```python
from build123d import *

# Parameters (mm, degrees)
CROQUIS2_R                    = 2.0193
CROQUIS2_R_2                  = 14.3256
CROQUIS2_R_3                  = 2.4892
SALIENTE_EXTRUIR1_DEPTH       = 6.35
CROQUIS4_R                    = 11.1125
CROQUIS4_R_2                  = 2.0193
CROQUIS4_R_3                  = 14.3256
CROQUIS4_R_4                  = 2.4892
CROQUIS4_R_5                  = 12.7
SALIENTE_EXTRUIR2_DEPTH       = 6.35
SALIENTE_EXTRUIR3_OUTLINE_R   = 2.4892
SALIENTE_EXTRUIR3_OUTLINE_R_2 = 11.1125
SALIENTE_EXTRUIR3_DEPTH       = 3.175


# Read off the part's stored shape, not the designer's step: Saliente-Extruir3
with BuildPart() as part:
    # Croquis2 → Saliente-Extruir1 (new body)
    with BuildSketch(Plane.XY):
        with BuildLine():
            Line((-50.26025, -3.966971602), (-17.216966667, -25.917547797))
            ThreePointArc((-17.216966667, -25.917547797), (0, -31.115), (17.216966667, -25.917547797))
            Line((17.216966667, -25.917547797), (50.26025, -3.966971602))
            ThreePointArc((50.26025, -3.966971602), (51.383179934, -2.925318757), (52.117388984, -1.581090594))
            Line((52.117388984, -1.581090594), (62.733042527, 28.581409406))
            ThreePointArc((62.733042527, 28.581409406), (59.824949243, 34.653759666), (53.750525482, 31.75))
            ThreePointArc((53.750525482, 31.75), (50.269530675, 27.147870067), (44.770269361, 25.4))
            Line((44.770269361, 25.4), (-44.770269361, 25.4))
            ThreePointArc((-44.770269361, 25.4), (-50.269530675, 27.147870067), (-53.750525482, 31.75))
            ThreePointArc((-53.750525482, 31.75), (-59.824949243, 34.653759666), (-62.733042527, 28.581409406))
            Line((-62.733042527, 28.581409406), (-52.117388984, -1.581090594))
            ThreePointArc((-52.117388984, -1.581090594), (-51.383179934, -2.925318757), (-50.26025, -3.966971602))
        make_face()
        with Locations((23.8125, 0)):
            Circle(CROQUIS2_R, mode=Mode.SUBTRACT)
        with Locations((-23.8125, 0)):
            Circle(CROQUIS2_R, mode=Mode.SUBTRACT)
        Circle(CROQUIS2_R_2, mode=Mode.SUBTRACT)
        with Locations((-47.625, 0)):
            Circle(CROQUIS2_R_3, mode=Mode.SUBTRACT)
        with Locations((47.625, 0)):
            Circle(CROQUIS2_R_3, mode=Mode.SUBTRACT)
        with Locations((-58.240653543, 30.1625)):
            Circle(CROQUIS2_R_3, mode=Mode.SUBTRACT)
        with Locations((58.240653543, 30.1625)):
            Circle(CROQUIS2_R_3, mode=Mode.SUBTRACT)
    extrude(amount=SALIENTE_EXTRUIR1_DEPTH)


with BuildPart() as body_2:
    # Croquis4 → Saliente-Extruir2 (new body)
    with BuildSketch(Plane.XY):
        with BuildLine():
            Line((-63.003153543, 56.9875), (-63.003153543, 30.1625))
            ThreePointArc((-63.003153543, 30.1625), (-62.935140138, 29.360501336), (-62.733042527, 28.581409406))
            Line((-62.733042527, 28.581409406), (-52.117388984, -1.581090594))
            ThreePointArc((-52.117388984, -1.581090594), (-51.383179934, -2.925318757), (-50.26025, -3.966971602))
            Line((-50.26025, -3.966971602), (-17.216966667, -25.917547797))
            ThreePointArc((-17.216966667, -25.917547797), (0, -31.115), (17.216966667, -25.917547797))
            Line((17.216966667, -25.917547797), (50.26025, -3.966971602))
            ThreePointArc((50.26025, -3.966971602), (51.383179934, -2.925318757), (52.117388984, -1.581090594))
            Line((52.117388984, -1.581090594), (62.733042527, 28.581409406))
            ThreePointArc((62.733042527, 28.581409406), (62.935140138, 29.360501336), (63.003153543, 30.1625))
            Line((63.003153543, 30.1625), (63.003153543, 56.9875))
            ThreePointArc((63.003153543, 56.9875), (54.216356978, 78.200703436), (33.003153543, 86.9875))
            Line((33.003153543, 86.9875), (-33.003153543, 86.9875))
            ThreePointArc((-33.003153543, 86.9875), (-54.216356978, 78.200703436), (-63.003153543, 56.9875))
        make_face()
        with Locations((0, 40.64)):
            Circle(CROQUIS4_R, mode=Mode.SUBTRACT)
        with Locations((-16.145831218, -9.3218)):
            Circle(CROQUIS4_R_2, mode=Mode.SUBTRACT)
        Circle(CROQUIS4_R_3, mode=Mode.SUBTRACT)
        with Locations((0, 18.6436)):
            Circle(CROQUIS4_R_2, mode=Mode.SUBTRACT)
        with Locations((16.145831218, -9.3218)):
            Circle(CROQUIS4_R_2, mode=Mode.SUBTRACT)
        with Locations((-47.625, 0)):
            Circle(CROQUIS4_R_4, mode=Mode.SUBTRACT)
        with Locations((47.625, 0)):
            Circle(CROQUIS4_R_4, mode=Mode.SUBTRACT)
        with Locations((-29.02971813, 82.074783851)):
            Circle(CROQUIS4_R_4, mode=Mode.SUBTRACT)
        with Locations((-36.976588955, 31.900216149)):
            Circle(CROQUIS4_R_4, mode=Mode.SUBTRACT)
        with Locations((-33.003153543, 56.9875)):
            Circle(CROQUIS4_R_5, mode=Mode.SUBTRACT)
        with Locations((-58.090437394, 60.960935412)):
            Circle(CROQUIS4_R_4, mode=Mode.SUBTRACT)
        with Locations((-58.240653543, 30.1625)):
            Circle(CROQUIS4_R_4, mode=Mode.SUBTRACT)
        with Locations((58.090437394, 60.960935412)):
            Circle(CROQUIS4_R_4, mode=Mode.SUBTRACT)
        with Locations((36.976588955, 31.900216149)):
            Circle(CROQUIS4_R_4, mode=Mode.SUBTRACT)
        with Locations((33.003153543, 56.9875)):
            Circle(CROQUIS4_R_5, mode=Mode.SUBTRACT)
        with Locations((29.02971813, 82.074783851)):
            Circle(CROQUIS4_R_4, mode=Mode.SUBTRACT)
        with Locations((58.240653543, 30.1625)):
            Circle(CROQUIS4_R_4, mode=Mode.SUBTRACT)
    extrude(amount=-SALIENTE_EXTRUIR2_DEPTH)


with BuildPart() as body_3:
    # Saliente-Extruir3 outline → Saliente-Extruir3 (new body)
    with BuildSketch(Plane.XY):
        with BuildLine():
            Line((-35.881109014, 27.265420582), (-22.987624276, 30.312923688))
            ThreePointArc((-22.987624276, 30.312923688), (-18.059295743, 30.166513899), (-13.86444293, 27.575555036))
            ThreePointArc((-13.86444293, 27.575555036), (0, 21.59), (13.86444293, 27.575555036))
            ThreePointArc((13.86444293, 27.575555036), (18.059295743, 30.166513899), (22.987624276, 30.312923688))
            Line((22.987624276, 30.312923688), (35.881109014, 27.265420582))
            ThreePointArc((35.881109014, 27.265420582), (41.611384522, 30.804736208), (38.072068895, 36.535011716))
            Line((38.072068895, 36.535011716), (23.323178626, 40.021058337))
            ThreePointArc((23.323178626, 40.021058337), (20.26820543, 41.736288231), (18.58786391, 44.81058932))
            ThreePointArc((18.58786391, 44.81058932), (18.032030897, 46.783969542), (17.267348762, 48.686189579))
            ThreePointArc((17.267348762, 48.686189579), (16.412494406, 53.542019269), (18.100083663, 58.174718315))
            Line((18.100083663, 58.174718315), (32.93018787, 79.342066878))
            ThreePointArc((32.93018787, 79.342066878), (31.762435104, 85.975253591), (25.129248391, 84.807500825))
            Line((25.129248391, 84.807500825), (11.314654439, 65.08961339))
            ThreePointArc((11.314654439, 65.08961339), (6.613405383, 61.027851685), (0.54804108, 59.682115192))
            ThreePointArc((0.54804108, 59.682115192), (0, 59.69), (-0.54804108, 59.682115192))
            ThreePointArc((-0.54804108, 59.682115192), (-6.613405383, 61.027851685), (-11.314654439, 65.08961339))
            Line((-11.314654439, 65.08961339), (-25.129248391, 84.807500825))
            ThreePointArc((-25.129248391, 84.807500825), (-31.762435104, 85.975253591), (-32.93018787, 79.342066878))
            Line((-32.93018787, 79.342066878), (-18.100083663, 58.174718315))
            ThreePointArc((-18.100083663, 58.174718315), (-16.412494406, 53.542019269), (-17.267348762, 48.686189579))
            ThreePointArc((-17.267348762, 48.686189579), (-18.032030897, 46.783969542), (-18.58786391, 44.81058932))
            ThreePointArc((-18.58786391, 44.81058932), (-20.26820543, 41.736288231), (-23.323178626, 40.021058337))
            Line((-23.323178626, 40.021058337), (-38.072068895, 36.535011716))
            ThreePointArc((-38.072068895, 36.535011716), (-41.611384522, 30.804736208), (-35.881109014, 27.265420582))
        make_face()
        with Locations((-36.976588955, 31.900216149)):
            Circle(SALIENTE_EXTRUIR3_OUTLINE_R, mode=Mode.SUBTRACT)
        with Locations((36.976588955, 31.900216149)):
            Circle(SALIENTE_EXTRUIR3_OUTLINE_R, mode=Mode.SUBTRACT)
        with Locations((0, 40.64)):
            Circle(SALIENTE_EXTRUIR3_OUTLINE_R_2, mode=Mode.SUBTRACT)
        with Locations((-29.02971813, 82.074783851)):
            Circle(SALIENTE_EXTRUIR3_OUTLINE_R, mode=Mode.SUBTRACT)
        with Locations((29.02971813, 82.074783851)):
            Circle(SALIENTE_EXTRUIR3_OUTLINE_R, mode=Mode.SUBTRACT)
    extrude(amount=SALIENTE_EXTRUIR3_DEPTH)


solid = part.part
```
Design review of the part built by this model. Coordinates are the model's own, in mm. A direction names the side the tool comes from. Give positions to 0.01 mm unless a question says otherwise; leave off trailing zeros. Order: outer loops, then holes, each group sorted by start corner. A loop starts at its lowest first (then second) coordinate and runs counter-clockwise, first axis right, second up. Notation, with made-up numbers: (60.25, 52) -> (65.25, 52) arc R32 ccw to (65.25, 80) -> close; hole circle Ø7 at (86, -23). An arc over 180 degrees is marked (long way). Write each question's results on one line, items separated by ' | '. Start each with the question number.
Q1. Mouldability with a two-part tool opening along X and no side actions: class faces 3 (the flat face through (1, 25.4, 3)), 4 (the cylindrical face through (-59.726, 34.687, 3.131)), 5 (the flat face through (-1, 17, 0)), 6 (the cylindrical face through (-51.396, -2.908, 3.131)) as +X half, -X half, draft (parallel to the pull), parting line (faces both ways), or undercut.
Q2. Add section C-C on y = 0. Give the boundary of the cut face in (x, z).
Q3. Add section A-A on x = 0. Give the boundary of the cut face in (y, z) (3 decimals).
Q4. Add section B-B on y = 12. Give the boundary of the cut face in (x, z), and give its area (3 significant figures).
Q5. Add section D-D on z = 4.75. State how many separate pieces and enclosed holes the cut face has, and give its area (3 significant figures).
Q6. Machinability: for faces 1 (the flat face through (57.35, 13.29, 3.13)), 2 (the cylindrical face through (50.34, 27.2, 3.13)), which of the approach directions +Z, -Z, +X, -X, +Y, -Y give a long, thin tool a straight path to every point of the face, cutting with its end or side? Answer none if there is none.
Q7. Wall thickness on L1, parallel to Y at x = -4.5, z = 1; L2, parallel to X at y = -5, z = 3.75; L3, parallel to Y at x = -46.5, z = 3.5: over which ranges is each line inside the solid? List them lowest first. Write a range as from..to.
Q8. For pin 1 (3 mm diameter, centred on x = -12.5, z = 4.5, fed in from +Y); pin 2 (8 mm diameter, centred on x = 58.24, y = 30.16, fed in from -Z); pin 3 (1.5 mm diameter, centred on y = -19, z = 5.5, fed in from -X), all flat-tipped, find the tip position at first contact; note any pin that passes through.
Found:
1) face 3: undercut | face 4: undercut | face 5: draft | face 6: -X half
2) outline: (-52.67, 0) -> (-50.11, 0) -> (-50.11, 6.35) -> (-52.67, 6.35) -> close; (-45.14, 0) -> (-25.83, 0) -> (-25.83, 6.35) -> (-45.14, 6.35) -> close; (-21.79, 0) -> (-14.33, 0) -> (-14.33, 6.35) -> (-21.79, 6.35) -> close; (14.33, 0) -> (21.79, 0) -> (21.79, 6.35) -> (14.33, 6.35) -> close; (25.83, 0) -> (45.14, 0) -> (45.14, 6.35) -> (25.83, 6.35) -> close; (50.11, 0) -> (52.67, 0) -> (52.67, 6.35) -> (50.11, 6.35) -> close
3) outline: (-31.115, 0) -> (-14.326, 0) -> (-14.326, 6.35) -> (-31.115, 6.35) -> close; (14.326, 0) -> (25.4, 0) -> (25.4, 6.35) -> (14.326, 6.35) -> close
4) outline: (-56.9, 0) -> (-7.82, 0) -> (-7.82, 6.35) -> (-56.9, 6.35) -> close; (7.82, 0) -> (56.9, 0) -> (56.9, 6.35) -> (7.82, 6.35) -> close | area: 623 mm2
5) separate pieces: 1 | enclosed holes: 7 | area: 4,350 mm2
6) face 1: +Z, -Z, +X, -Y | face 2: +Z, -Z, +Y
7) L1: y = -30.79..-13.6, 13.6..25.4 | L2: x = -48.71..-13.42, 13.42..48.71 | L3: y = -6.46..-2.22, 2.22..25.56
8) pin 1: stops at y = 25.4 | pin 2: stops at z = 0 | pin 3: stops at x = -28.76
